The model under review builds one solid part; all positions refer to its coordinate system, in mm. A direction names the side the tool comes from. Round coordinates to 2 decimals unless told otherwise and drop trailing zeros. Order: outer loops, then holes, each group sorted by start corner. A loop starts at its lowest first (then second) coordinate and runs counter-clockwise, first axis right, second up. Notation, with made-up numbers: M 49.5,-9 L 93.5,-9 A31 cw 93.5,15 Z; hole C 19,27 d10. An arc over 180 degrees is marked long. Answer as a JSON object with one key per item and string values. Group by question number.
1. Add section A-A on z = 0. State the section outline as (x, y) points (3 decimals), and give its area (3 significant figures).
2. Add section C-C on y = 2. Give the number of separate pieces and of enclosed holes in the cut face, and give its area (3 significant figures).
3. To check wall thickness, follow probe 1 along X at (y, z) = (2, -0.5) (3 decimals); probe 2 along X at (y, z) = (0.5, -8) (1 decimal); probe 3 along Z at (x, y) = (-126, 2). State the ranges of each line that lie inside material, in increasing order. Write a range as [from, to].
4. Clearance check with flat-ended pins moving along their axes: P1, Ø3, axis at x = -112.5, y = 2, coming from the +Z side; P2, Ø3.5, axis at x = 40.56, z = -53.19, coming from the +Y side; P3, Ø1.5, axis at x = -119, y = 1, coming from the -Z side; P4, Ø3, axis at x = -102, y = 3, coming from the +Z side. State where each tip first meets the part, or that it passes through.
5. Machinability: for faces 1 (the face through (45.45, 3.22, 61.21)), 2 (the face through (-65, 3.13, -7.78)), which of the approach directions +Z, -Z, +X, -X, +Y, -Y give a long, thin tool a straight path to every point of the face, cutting with its end or side? Answer none if there is none.
6. Mouldability with a two-part tool opening along Z and no side actions: class faces 3 (the face through (-4, 3, 63.5)), 4 (the face through (-189.658, 3.219, -0.45)), 5 (the face through (-63.5, 3, -24)) as released by +Z, released by -Z, zero draft, split by the parting line, or undercut.
7. Add section D-D on z = 40. State the section outline as (x, y) points (3 decimals), and give its area (3 significant figures).
8. Add section B-B on x = -76. State the section outline as (y, z) points.
```python
from build123d import *

# Parameters (mm, degrees)
SKETCH1_W           = 95.25
SKETCH1_H           = 127
BOSS_EXTRUDE1_DEPTH = 6.35
BOSS_EXTRUDE3_DEPTH = 6.35
SKETCH5_R           = 4.826
SKETCH5_R_2         = 2.5
SKETCH5_R_3         = 1.5
CUT_EXTRUDE1_DEPTH  = 7.35
CUT_EXTRUDE2_DEPTH  = 7.35
FILLET9_R           = 5
FILLET10_R          = 7.62
SKETCH7_R           = 2.2812375
CUT_EXTRUDE3_DEPTH  = 7.35
SKETCH8_R           = 1.830008083
CUT_EXTRUDE4_DEPTH  = 7.35


with BuildPart() as part:
    # Sketch1 → Boss-Extrude1 (new body)
    with BuildSketch(Plane(origin=(0, 0, 0), x_dir=(1, 0, 0), z_dir=(0, 1, 0))):
        Rectangle(SKETCH1_W, SKETCH1_H)
    extrude(amount=BOSS_EXTRUDE1_DEPTH)

    # Sketch4 → Boss-Extrude3 (add)
    with BuildSketch(Plane(origin=(0, 6.35, 0), x_dir=(1, 0, 0), z_dir=(0, 1, 0))):
        with BuildLine():
            Line((-47.625, 63.5), (-171.916018217, 24.219268021))
            ThreePointArc((-171.916018217, 24.219268021), (-189.6618, 0), (-171.916018217, -24.219268021))
            Line((-171.916018217, -24.219268021), (-47.625, -63.5))
            Line((-47.625, -63.5), (-47.625, 63.5))
        make_face()
    extrude(amount=-BOSS_EXTRUDE3_DEPTH)

    # Sketch5 → Cut-Extrude1 (cut, through all)
    with BuildSketch(Plane(origin=(0, 6.35, 0), x_dir=(1, 0, 0), z_dir=(0, 1, 0))):
        with Locations((-164.2618, 0)):
            Circle(SKETCH5_R)
        with Locations((-48.9458, 0)):
            Circle(SKETCH5_R_2)
        with Locations((-40.106965235, 8.838834765)):
            Circle(SKETCH5_R_3)
        with Locations((-57.784634765, -8.838834765)):
            Circle(SKETCH5_R_3)
        with Locations((-55.663314421, 6.717514421)):
            Circle(SKETCH5_R_3)
        with Locations((-42.228285579, -6.717514421)):
            Circle(SKETCH5_R_3)
    extrude(amount=-CUT_EXTRUDE1_DEPTH, mode=Mode.SUBTRACT)

    # Sketch6 → Cut-Extrude2 (cut, through all)
    with BuildSketch(Plane(origin=(0, 6.35, 0), x_dir=(1, 0, 0), z_dir=(0, 1, 0))):
        Polygon((-63.5, 45.163743355), (-157.9118, 6.35), (-63.5, 6.35), align=None)
        Polygon((-63.5, -6.35), (-63.5, -45.163743355), (-157.9118, -6.35), align=None)
    extrude(amount=-CUT_EXTRUDE2_DEPTH, mode=Mode.SUBTRACT)

    # Fillet9
    fillet9_edges = [part.edges().sort_by_distance(p)[0] for p in [
        (-63.5, 3.175, -45.163743355),
        (-63.5, 3.175, -6.35),
        (-157.9118, 3.175, -6.35),
        (-157.9118, 3.175, 6.35),
        (-63.5, 3.175, 6.35),
        (-63.5, 3.175, 45.163743355),
    ]]
    fillet(fillet9_edges, radius=FILLET9_R)

    # Fillet10
    fillet10_edges = [part.edges().sort_by_distance(p)[0] for p in [
        (47.625, 3.175, 63.5),
        (47.625, 3.175, -63.5),
    ]]
    fillet(fillet10_edges, radius=FILLET10_R)

    # Sketch7 → Cut-Extrude3 (cut, through all)
    with BuildSketch(Plane(origin=(0, 6.35, 0), x_dir=(1, 0, 0), z_dir=(0, 1, 0))):
        with Locations((-46.889614099, -53.200246229)):
            Circle(SKETCH7_R)
        with Locations((-46.889614099, 53.180131976)):
            Circle(SKETCH7_R)
        with Locations((40.557033552, 53.190189103)):
            Circle(SKETCH7_R)
        with Locations((40.539614099, -53.220360481)):
            Circle(SKETCH7_R)
    extrude(amount=-CUT_EXTRUDE3_DEPTH, mode=Mode.SUBTRACT)

    # Sketch8 → Cut-Extrude4 (cut, through all)
    with BuildSketch(Plane(origin=(0, 6.35, 0), x_dir=(1, 0, 0), z_dir=(0, 1, 0))):
        with Locations((-6.328465047, -19.828924843)):
            Circle(SKETCH8_R)
        with Locations((-6.328338046, 21.171490961)):
            Circle(SKETCH8_R)
    extrude(amount=-CUT_EXTRUDE4_DEPTH, mode=Mode.SUBTRACT)


solid = part.part
```
Recorded:
{
 "1": {"outline": "M -189.662,0 L -169.088,0 L -169.088,6.35 L -189.662,6.35 Z; M -159.436,0 L -51.446,0 L -51.446,6.35 L -159.436,6.35 Z; M -46.446,0 L 47.625,0 L 47.625,6.35 L -46.446,6.35 Z", "area": "1,410 mm²"},
 "2": {"separate pieces": "1", "enclosed holes": "14", "area": "20,000 mm²"},
 "3": {"probe 1": "x = [-189.657, -169.062], [-159.462, -51.395], [-46.496, 47.625]", "probe 2": "x = [-188.4, -136.3], [-64.8, -56.4], [-54.9, -41.4], [-38.9, 47.6]", "probe 3": "z = [-38.73, -19.47], [-6.35, 6.35], [19.47, 38.73]"},
 "4": {"P1": "stops at z = 43.47", "P2": "passes through", "P3": "stops at z = -41.18", "P4": "stops at z = 46.79"},
 "5": {"face 1": "+Z, +X, +Y, -Y", "face 2": "+Y, -Y"},
 "6": {"face 3": "released by +Z", "face 4": "split by the parting line", "face 5": "undercut"},
 "7": {"outline": "M -121.983,0 L -76.06,0 L -76.06,6.35 L -121.983,6.35 Z; M -64.059,0 L 47.625,0 L 47.625,6.35 L -64.059,6.35 Z", "area": "1,000 mm²"},
 "8": {"outline": "M 0,-54.53 L 6.35,-54.53 L 6.35,-40.02 L 0,-40.02 Z; M 0,-6.35 L 6.35,-6.35 L 6.35,6.35 L 0,6.35 Z; M 0,40.02 L 6.35,40.02 L 6.35,54.53 L 0,54.53 Z"}
}
